Geometry: final body of the model. Coordinates: model frame, mm. A direction names the side the tool comes from. Give positions to 0.01 mm unless a question says otherwise; leave off trailing zeros. Write each loop counter-clockwise with the first axis right and the second up, starting at its lowest first coordinate (ties: lowest second). Pieces come first, ordered by that corner, then holes. Notation, with made-up numbers: M -4,30 L 36,30 A24 cw 36,54 Z; hole C 16.25,-5.75 d7. An arc over 180 degrees is marked long. Use one line per item in the form item = value. Start each with the question number.
Item 1: Pull-direction query (X, two-part tool) for faces 1 (the flat face through (-35, -13.5, 1)), 2 (the flat face through (50, -10, 1)); classes: released by +X, released by -X, zero draft, split by the parting line, or undercut.
Item 2: Section query A-A on x = -14.5. Return loops of the section in (y, z), then the cut area to 3 significant figures.
Item 3: Contact query for flat-ended pins moving along their axis: P1, Ø1.5, axis at x = -1.5, z = 1, coming from the +Y side; P2, Ø1.5, axis at y = -9, z = 1, coming from the -X side; P3, Ø8, axis at x = 8.5, y = 7, coming from the -Z side; P4, Ø0.9, axis at y = -8.5, z = 2, coming from the +X side. Output: stop coordinate, or through.
Item 4: Material intervals for line 1 along X through (y, z) = (-8.75, 2.5); line 2 along X through (y, z) = (8, 1.8); line 3 along Y through (x, z) = (1, 0.35), sorted ascending. Write a range as from..to.
Item 5: Section query B-B on y = 8.5. Return loops of the section in (x, z).
Item 6: Section query C-C on z = 1.5. Give the number of separate pieces and of enclosed holes in the cut face, then the cut area to 3 significant figures.
Item 7: Access query for faces 3 (the flat face through (-51, 7, 1)), 4 (the flat face through (35, -13.5, 1)). Directions: +Z, -Z, +X, -X, +Y, -Y. A direction counts if a zero-diameter tool reaches every point of the face in a straight line with its end or side. Return the directions, or none.
Autodesk Inventor part; units mm, degrees
ref_plane "YZ Plane" through (0, 0, 0) normal (1, 0, 0) x (0, 1, 0)
ref_plane "XZ Plane" through (0, 0, 0) normal (0, 1, 0) x (-1, 0, 0)
ref_plane "XY Plane" through (0, 0, 0) normal (0, 0, 1) x (1, 0, 0)
sketch "Esboço1" plane through (0, 0, 0) normal (0, 0, 1) x (1, 0, 0)
  arc A0 (-63, 13.5) -> (-75, 0) centre (-61.4063, 0) ccw
  line L0 (0, 10) -> (-3.5, 10)
  arc A1 (-5.25, 11.75) -> (-7, 13.5) centre (-7, 11.75) ccw
  arc A2 (-5.25, 11.75) -> (-3.5, 10) centre (-3.5, 11.75) ccw
  line L1 (-7, 13.5) -> (-63, 13.5)
  line L2 (-49, 10) -> (-52, 10)
  line L3 (-52, 10) -> (-52, 7)
  line L4 (-52, 7) -> (-49, 7)
  line L5 (-49, 7) -> (-49, 10)
  line L6 (-13, 10) -> (-16, 10)
  line L7 (-16, 10) -> (-16, 7)
  line L8 (-16, 7) -> (-13, 7)
  line L9 (-13, 7) -> (-13, 10)
  line L10 (0, 10) -> (3.5, 10)
  arc A3 (3.5, 10) -> (5.25, 11.75) centre (3.5, 11.75) ccw
  arc A4 (7, 13.5) -> (5.25, 11.75) centre (7, 11.75) ccw
  line L11 (7, 13.5) -> (63, 13.5)
  arc A5 (75, 0) -> (63, 13.5) centre (61.4063, 0) ccw
  line L12 (49, 10) -> (52, 10)
  line L13 (52, 10) -> (52, 7)
  line L14 (52, 7) -> (49, 7)
  line L15 (49, 7) -> (49, 10)
  line L16 (13, 10) -> (16, 10)
  line L17 (16, 10) -> (16, 7)
  line L18 (16, 7) -> (13, 7)
  line L19 (13, 7) -> (13, 10)
  line L20 (0, -10) -> (-3.5, -10)
  arc A6 (-3.5, -10) -> (-5.25, -11.75) centre (-3.5, -11.75) ccw
  arc A7 (-7, -13.5) -> (-5.25, -11.75) centre (-7, -11.75) ccw
  line L21 (-7, -13.5) -> (-63, -13.5)
  arc A8 (-75, 0) -> (-63, -13.5) centre (-61.4063, 0) ccw
  line L22 (-49, -10) -> (-52, -10)
  line L23 (-52, -10) -> (-52, -7)
  line L24 (-52, -7) -> (-49, -7)
  line L25 (-49, -7) -> (-49, -10)
  line L26 (-13, -10) -> (-16, -10)
  line L27 (-16, -10) -> (-16, -7)
  line L28 (-16, -7) -> (-13, -7)
  line L29 (-13, -7) -> (-13, -10)
  arc A9 (63, -13.5) -> (75, 0) centre (61.4063, 0) ccw
  line L30 (52, -10) -> (52, -7)
  line L31 (49, -10) -> (52, -10)
  line L32 (52, -7) -> (49, -7)
  line L33 (49, -7) -> (49, -10)
  line L34 (7, -13.5) -> (63, -13.5)
  line L35 (16, -10) -> (16, -7)
  line L36 (16, -7) -> (13, -7)
  line L37 (13, -10) -> (16, -10)
  line L38 (13, -7) -> (13, -10)
  arc A10 (5.25, -11.75) -> (7, -13.5) centre (7, -11.75) ccw
  arc A11 (5.25, -11.75) -> (3.5, -10) centre (3.5, -11.75) ccw
  line L39 (0, -10) -> (3.5, -10)
  point P0 (0, 0)
  dimension "d6" = 3.5
extrude "Extrusão1" add sketch "Esboço1" along normal blind 3
properties part number "ASA_SUPERIOR"
Answer sheet:
q1.face_1 = zero draft
q1.face_2 = undercut
q2.outline = M -13.5,0 L -10,0 L -10,3 L -13.5,3 Z; M -7,0 L 7,0 L 7,3 L -7,3 Z; M 10,0 L 13.5,0 L 13.5,3 L 10,3 Z
q2.area = 63.0 mm2
q3.P1 = 10
q3.P2 = -72.21
q3.P3 = 0
q3.P4 = 72.36
q4.line_1 = -71.81..-52, -49..-16, -13..13, 16..49, 52..71.81
q4.line_2 = -72.4..-52, -49..-16, -13..13, 16..49, 52..72.4
q4.line_3 = -10..10
q5.outline = M -72.01,0 L -52,0 L -52,3 L -72.01,3 Z; M -49,0 L -16,0 L -16,3 L -49,3 Z; M -13,0 L 13,0 L 13,3 L -13,3 Z; M 16,0 L 49,0 L 49,3 L 16,3 Z; M 52,0 L 72.01,0 L 72.01,3 L 52,3 Z
q6.separate_pieces = 1
q6.enclosed_holes = 8
q6.area = 3,750 mm2
q7.face_3 = +Z, -Z
q7.face_4 = +Z, -Z, +X, -X, -Y
